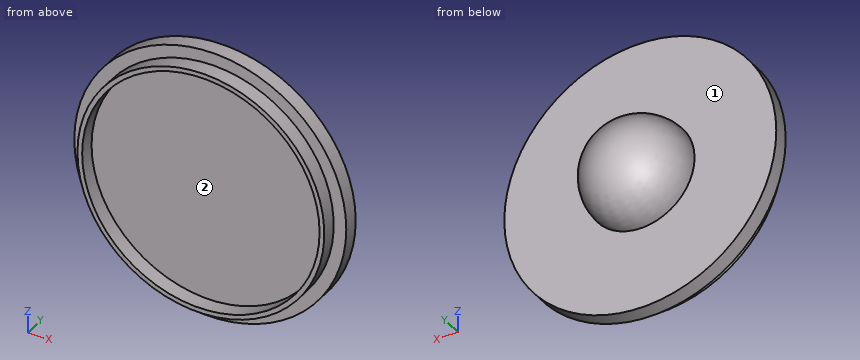
from build123d import *


with BuildPart() as part:
    # Croquis1 → Revolución1 (revolve)
    with BuildSketch(Plane.XY):
        with BuildLine():
            Line((-27.691646337, -4.777448071), (-27.691646337, -1.777448071))
            Line((-27.691646337, -1.777448071), (-4.991646337, -1.777448071))
            Line((-4.991646337, -1.777448071), (-4.991646337, 11.222551929))
            ThreePointArc((-4.991646337, 11.222551929), (-12.252224974, 8.372117695), (-15.370667987, 1.222551929))
            Line((-15.370667987, 1.222551929), (-30.991646337, 1.222551929))
            Line((-30.991646337, 1.222551929), (-30.991646337, -1.777448071))
            Line((-30.991646337, -1.777448071), (-28.591646337, -1.777448071))
            Line((-28.591646337, -1.777448071), (-28.591646337, -4.777448071))
            Line((-28.591646337, -4.777448071), (-27.691646337, -4.777448071))
        make_face()
    revolve(axis=Axis((-4.991646337, 5.975396892, 0), (0, -1, 0)))


solid = part.part
Source: CAD feature listing. Evaluate the final solid. Frame: model axes, mm. Face numbers are marked on the shaded views. Round coordinates to 2 decimals unless told otherwise and drop trailing zeros. Order: outer loops, then holes, each group sorted by start corner. A loop starts at its lowest first (then second) coordinate and runs counter-clockwise, first axis right, second up. Notation, with made-up numbers: (71, -37) -> (123, -37) arc R14 cw to (123, -25) -> close; hole circle Ø6 at (-3.5, 13.5). An arc over 180 degrees is marked (long way). Answer as CSV lines item,"result".
Item 1: Pull-direction query (X, two-part tool) for the marked faces 1 and 2; classes: pulls with the +X half, pulls with the -X half, needs draft (parallel to the pull), parting line crosses it, or undercut.
A:
face 1,"needs draft"
face 2,"undercut"
Item 2: Section B-B, the plane x = -22. Return loops of the section in (y, z).
A:
outline,"(-4.78, -16.36) -> (-1.78, -16.36) -> (-1.78, -19.67) -> (1.22, -19.67) -> (1.22, 19.67) -> (-1.78, 19.67) -> (-1.78, 16.36) -> (-4.78, 16.36) -> (-4.78, 15.03) -> (-1.78, 15.03) -> (-1.78, -15.03) -> (-4.78, -15.03) -> close"
Item 3: Section A-A, the plane z = 16. Return loops of the section in (x, y).
A:
outline,"(-25.49, -1.78) -> (-22.34, -1.78) -> (-22.34, -4.78) -> (-21.09, -4.78) -> (-21.09, -1.78) -> (11.11, -1.78) -> (11.11, -4.78) -> (12.36, -4.78) -> (12.36, -1.78) -> (15.5, -1.78) -> (15.5, 1.22) -> (-25.49, 1.22) -> close"
Item 4: Line query: L1, parallel to X at y = -3.2, z = 0; L2, parallel to Y at x = 10, z = -5.5; L3, parallel to Z at x = -17.5, y = -3. Output: solid intervals per line, ascending.
A:
L1,"-28.59 to -27.69, 17.71 to 18.61"
L2,"-1.78 to 1.22"
L3,"-20.01 to -18.94, 18.94 to 20.01"
Item 5: Pin query (flat end, axial travel): pin 1 Ø12 at (x, z) = (-3.5, 10.5) entering from -Y; pin 2 Ø8 at (x, y) = (-21, -1.5) entering from +Z; pin 3 Ø4 at (x, z) = (-2, 6) entering from +Y; pin 4 Ø2 at (x, y) = (15.5, 4) entering from +Z. Return the tip coordinate at first contact, or that it passes through.
A:
pin 1,"y = -1.78"
pin 2,"z = 23.06"
pin 3,"y = 10.17"
pin 4,"through"
